Source: CAD feature listing. Evaluate the final solid. Frame: model axes, mm. Face numbers are marked on the shaded views. A direction names the side the tool comes from. Round coordinates to 2 decimals unless told otherwise and drop trailing zeros. Loops run counter-clockwise (first coordinate to the right, second up) from the corner with the lowest first, then second, coordinate; pieces in that order, holes last. Notation, with made-up numbers: (-34.5, 79) - (-6.5, 79) arc R37 cw to (-6.5, 115) - close; hole circle Ø2 at (6, -0.75). An arc over 180 degrees is marked (long way). One line per question, with ' | ' between items. Start each with the question number.
1. Mould query, pull axis X, two halves, no side actions, for the marked faces 6, 7, 8 and 9. Classes: pulls with the +X half, pulls with the -X half, needs draft (parallel to the pull), parting line crosses it, or undercut.
2. Cut plane B-B (y = 67.5). Return loops of the section in (x, z).
3. Access query for the marked faces 1, 2, 3, 4 and 5. Directions: +Z, -Z, +X, -X, +Y, -Y. A direction counts if a zero-diameter tool reaches every point of the face in a straight line with its end or side. Return the directions, or none.
4. Ray query, line 1 (Y direction, x = 351, z = 316.5); line 2 (X direction, y = 586.5, z = 290.5); line 3 (Z direction, x = 146.5, y = 546.5). Return the intervals inside material, ascending.
5. Cut plane A-A (x = 106). Return loops of the section in (y, z).
6. Cut plane C-C (z = 39.5). Return loops of the section in (x, y).
```python
from build123d import *

# Parameters (mm, degrees)
CROQUIS1_W              = 450
CROQUIS1_H              = 620
SALIENTE_EXTRUIR1_DEPTH = 350
CROQUIS2_W              = 390
CROQUIS2_H              = 80
CORTAR_EXTRUIR1_DEPTH   = 350
CROQUIS3_W              = 390
CROQUIS3_H              = 110
CORTAR_EXTRUIR2_DEPTH   = 350
SALIENTE_EXTRUIR2_DEPTH = 420


with BuildPart() as part:
    # Croquis1 → Saliente-Extruir1 (new body)
    with BuildSketch(Plane.XY):
        with Locations((225, 310)):
            Rectangle(CROQUIS1_W, CROQUIS1_H)
    extrude(amount=SALIENTE_EXTRUIR1_DEPTH)

    # Croquis2 → Cortar-Extruir1 (cut)
    with BuildSketch(Plane.XY.offset(350)):
        with Locations((225, 40)):
            Rectangle(CROQUIS2_W, CROQUIS2_H)
    extrude(amount=-CORTAR_EXTRUIR1_DEPTH, mode=Mode.SUBTRACT)

    # Croquis3 → Cortar-Extruir2 (cut)
    with BuildSketch(Plane.XY.offset(350)):
        with Locations((225, 535)):
            Rectangle(CROQUIS3_W, CROQUIS3_H)
    extrude(amount=-CORTAR_EXTRUIR2_DEPTH, mode=Mode.SUBTRACT)

    # Croquis4 → Saliente-Extruir2 (add)
    with BuildSketch(Plane(origin=(30, 0, 0), x_dir=(0, 0, -1), z_dir=(1, 0, 0))):
        Polygon((-350, 480), (-320.882381259, 560), (-29.117618741, 560), (0, 480), (0, 453.27353989), (-350, 453.27353989), align=None)
    extrude(amount=SALIENTE_EXTRUIR2_DEPTH)


solid = part.part
```
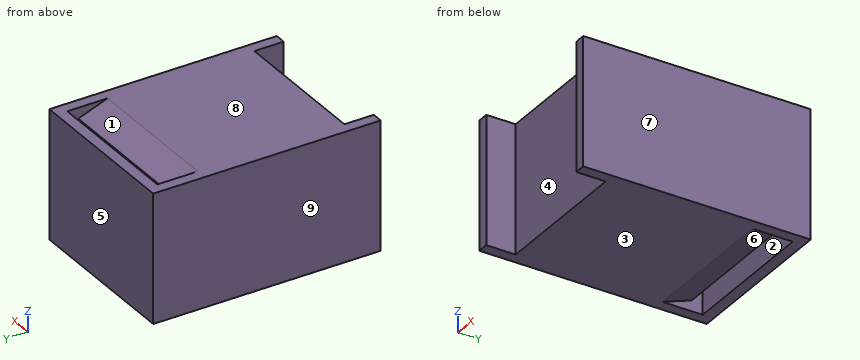
Answers follow:
1) face 6: undercut | face 7: pulls with the +X half | face 8: needs draft | face 9: pulls with the -X half
2) outline: (0, 0) - (30, 0) - (30, 350) - (0, 350) - close; (420, 0) - (450, 0) - (450, 350) - (420, 350) - close
3) face 1: +Z | face 2: +Z, -Z | face 3: -Z, +X, -X, +Y, -Y | face 4: +Z, -Z, -Y | face 5: +Z, -Z, +X, -X, +Y
4) line 1: y = 80 to 560, 590 to 620 | line 2: x = 0 to 30, 420 to 450 | line 3: z = 24.2 to 325.8
5) outline: (80, 0) - (480, 0) - (560, 29.12) - (560, 320.88) - (480, 350) - (80, 350) - close; (590, 0) - (620, 0) - (620, 350) - (590, 350) - close
6) outline: (0, 0) - (30, 0) - (30, 80) - (420, 80) - (420, 0) - (450, 0) - (450, 620) - (0, 620) - close; hole (30, 560) - (420, 560) - (420, 590) - (30, 590) - close
